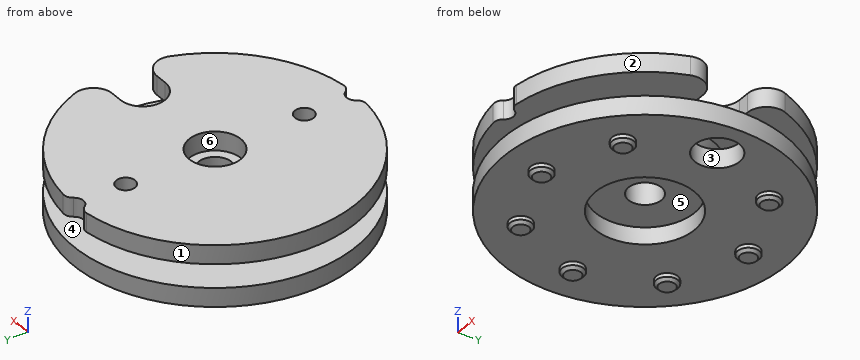
from build123d import *

# Parameters (mm, degrees)
SKETCH1_R                       = 15
BODY_DEPTH                      = 3.25
SKETCH2_R                       = 15
SKETCH2_R_2                     = 6.5
PULLEY_CLEARANCE_DEPTH          = 1.25
SKETCH3_R                       = 1.75
MAIN_BOLT_THROUGH_HOLE_DEPTH    = 7.5
SKETCH4_R                       = 5.25
SERVO_HORN_CLEARANCE_DEPTH      = 1.8
SKETCH5_R                       = 2.75
MAIN_BOLT_CLEARANCE_DEPTH       = 2
SKETCH6_R                       = 2.375
HORN_ATTACHMENT_HOLES_DEPTH     = 7.5
HORN_ATTACHMENT_CLEARANCE_DEPTH = 2
SKETCH8_R                       = 1
TENDON_ANCHOR_DEPTH             = 2
CONTOURING_BOLT_R               = 2
INNER_CHAMFER_SIZE              = 0.75
CONTOURING_TENDON_R             = 1
SKETCH9_R                       = 1.15
LOCKING_NUBS_DEPTH              = 0.7
NUB_CHAMFERS_SIZE               = 0.3


with BuildPart() as part:
    # Sketch1 → Body (new body, symmetric)
    with BuildSketch(Plane.XY):
        Circle(SKETCH1_R)
    extrude(amount=BODY_DEPTH, both=True)

    # Sketch2 → Pulley Clearance (cut, symmetric)
    with BuildSketch(Plane.XY):
        Circle(SKETCH2_R)
        Circle(SKETCH2_R_2, mode=Mode.SUBTRACT)
    extrude(amount=PULLEY_CLEARANCE_DEPTH, both=True, mode=Mode.SUBTRACT)

    # Sketch3 → Main Bolt Through Hole (cut, through all)
    with BuildSketch(Plane.XY.offset(3.25)):
        Circle(SKETCH3_R)
    extrude(amount=-MAIN_BOLT_THROUGH_HOLE_DEPTH, mode=Mode.SUBTRACT)

    # Sketch4 → Servo Horn Clearance (cut)
    with BuildSketch(Plane(origin=(0, 0, -3.25), x_dir=(-1, 0, 0), z_dir=(0, 0, -1))):
        Circle(SKETCH4_R)
    extrude(amount=-SERVO_HORN_CLEARANCE_DEPTH, mode=Mode.SUBTRACT)

    # Sketch5 → Main Bolt Clearance (cut)
    with BuildSketch(Plane.XY.offset(3.25)):
        Circle(SKETCH5_R)
    extrude(amount=-MAIN_BOLT_CLEARANCE_DEPTH, mode=Mode.SUBTRACT)

    # Sketch6 → Horn Attachment Holes (cut, through all)
    with BuildSketch(Plane(origin=(0, 0, -3.25), x_dir=(-1, 0, 0), z_dir=(0, 0, -1))):
        with Locations((-11, 0)):
            Circle(SKETCH6_R)
    extrude(amount=-HORN_ATTACHMENT_HOLES_DEPTH, mode=Mode.SUBTRACT)

    # Sketch7 → Horn Attachment Clearance (cut)
    with BuildSketch(Plane.XY.offset(3.25)):
        with BuildLine():
            Line((11, -2.375), (11, 2.375))
            Line((11, 2.375), (14.810785766, 2.375))
            ThreePointArc((14.810785766, 2.375), (15, 0), (14.810785766, -2.375))
            Line((14.810785766, -2.375), (11, -2.375))
        make_face()
    extrude(amount=-HORN_ATTACHMENT_CLEARANCE_DEPTH, mode=Mode.SUBTRACT)

    # Sketch8 → Tendon Anchor (cut)
    with BuildSketch(Plane.XY.offset(3.25)):
        with Locations((0, 9.5)):
            Circle(SKETCH8_R)
        with Locations((0, 15)):
            Circle(SKETCH8_R)
        with Locations((0, -15)):
            Circle(SKETCH8_R)
        with Locations((0, -9.5)):
            Circle(SKETCH8_R)
    extrude(amount=-TENDON_ANCHOR_DEPTH, mode=Mode.SUBTRACT)

    # Contouring - Bolt
    contouring_bolt_edges = [part.edges().sort_by_distance(p)[0] for p in [
        (14.810785766, -2.375, 2.25),
        (14.810785766, 2.375, 2.25),
    ]]
    fillet(contouring_bolt_edges, radius=CONTOURING_BOLT_R)

    # Inner Chamfer
    inner_chamfer_edges = [part.edges().sort_by_distance(p)[0] for p in [
        (-6.5, 0, -1.25),
        (-6.5, 0, 1.25),
    ]]
    chamfer(inner_chamfer_edges, length=INNER_CHAMFER_SIZE)

    # Contouring - Tendon
    contouring_tendon_edges = [part.edges().sort_by_distance(p)[0] for p in [
        (-0.99944429, 14.966666667, 2.25),
        (0.99944429, 14.966666667, 2.25),
        (0.99944429, -14.966666667, 2.25),
        (-0.99944429, -14.966666667, 2.25),
    ]]
    fillet(contouring_tendon_edges, radius=CONTOURING_TENDON_R)

    # Sketch9 → Locking Nubs (add)
    with BuildSketch(Plane(origin=(0, 0, -3.25), x_dir=(-1, 0, 0), z_dir=(0, 0, -1))):
        with Locations((11, 0)):
            Circle(SKETCH9_R)
        with Locations((7.778174593, -7.778174593)):
            Circle(SKETCH9_R)
        with Locations((0, -11)):
            Circle(SKETCH9_R)
        with Locations((-7.778174593, -7.778174593)):
            Circle(SKETCH9_R)
        with Locations((-7.778174593, 7.778174593)):
            Circle(SKETCH9_R)
        with Locations((0, 11)):
            Circle(SKETCH9_R)
        with Locations((7.778174593, 7.778174593)):
            Circle(SKETCH9_R)
    extrude(amount=LOCKING_NUBS_DEPTH)

    # Nub Chamfers
    nub_chamfers_edges = [part.edges().sort_by_distance(p)[0] for p in [
        (-9.85, 0, -3.95),
        (-6.628174593, -7.778174593, -3.95),
        (1.15, -11, -3.95),
        (8.928174593, -7.778174593, -3.95),
        (8.928174593, 7.778174593, -3.95),
        (1.15, 11, -3.95),
        (-6.628174593, 7.778174593, -3.95),
    ]]
    chamfer(nub_chamfers_edges, length=NUB_CHAMFERS_SIZE)


solid = part.part
Work out the finished part from the listing and answer in its coordinate system (mm). Face numbers are marked on the shaded views. A direction names the side the tool comes from. Round coordinates to 2 decimals unless told otherwise and drop trailing zeros. Write each loop counter-clockwise with the first axis right and the second up, starting at its lowest first coordinate (ties: lowest second). Pieces come first, ordered by that corner, then holes.
1) A cutting plane is placed at A-A (x = -11). Give the vertices of the cut face in (y, z).
2) Given pin 1 Ø2 at (x, z) = (-10, 2.5) entering from +Y; pin 2 Ø1.6 at (x, y) = (0.5, 0.5) entering from +Z; pin 3 Ø2 at (x, z) = (-3.5, -2) entering from -Y; pin 4 Ø1.4 at (x, z) = (11.5, 2) entering from +Y, each flat-ended and moving along its own axis, determine where each tip first touches the part or whether it passes through.
3) A cutting plane is placed at D-D (z = 2). Give the number of separate pieces and of enclosed holes in the cut face, plus the area to 3 significant figures.
4) A tool of negligible diameter and unlimited length cuts with its end or side. For the marked faces 4, 5 and 6, from which of +Z, -Z, +X, -X, +Y, -Y can it reach the whole face along a straight path? Write none if from no direction.
5) A cutting plane is placed at C-C (y = 9.5). Give the vertices of the cut face in (x, z).
6) The mould has two halves that part along X. Classify the marked faces 1, 2 and 3: pulls with the +X half, pulls with the -X half, needs draft (parallel to the pull), parting line crosses it, or undercut.
7) Straight lines are drawn through the part: line 1 (Z direction, x = -9, y = -0.5); line 2 (Z direction, x = 7.5, y = -8.25); line 3 (Y direction, x = 0, z = -2.1). For each, find the intervals that lie inside material, in ascending order.
Completed:
1. outline: (-10.2, -3.25) - (-1.15, -3.25) - (-1.15, -3.65) - (-0.85, -3.95) - (0.85, -3.95) - (1.15, -3.65) - (1.15, -3.25) - (10.2, -3.25) - (10.2, -1.25) - (-10.2, -1.25) - close; (-10.2, 1.25) - (10.2, 1.25) - (10.2, 3.25) - (-10.2, 3.25) - close
2. pin 1: stops at y = 12
2. pin 2: passes through
2. pin 3: stops at y = -14.79
2. pin 4: stops at y = 10.41
3. separate pieces: 1
3. enclosed holes: 3
3. area: 643 mm2
4. face 4: none
4. face 5: -Z
4. face 6: +Z
5. outline: (-11.61, -3.25) - (11.61, -3.25) - (11.61, -1.25) - (-11.61, -1.25) - close; (-11.61, 1.25) - (-1, 1.25) - (-1, 3.25) - (-11.61, 3.25) - close; (1, 1.25) - (11.61, 1.25) - (11.61, 3.25) - (1, 3.25) - close
6. face 1: pulls with the -X half
6. face 2: pulls with the +X half
6. face 3: undercut
7. line 1: z = -3.25 to -1.25, 1.25 to 3.25
7. line 2: z = -3.95 to -1.25, 1.25 to 3.25
7. line 3: y = -15 to -5.25, 5.25 to 15
